Here's how the part is built. I have some questions about the finished solid (model axes, mm). A direction names the side the tool comes from. Give positions to 0.01 mm unless a question says otherwise; leave off trailing zeros. Write each loop counter-clockwise with the first axis right and the second up, starting at its lowest first coordinate (ties: lowest second). Pieces come first, ordered by that corner, then holes. Notation, with made-up numbers: (3, -14) -> (53, -14) arc R21 cw to (53, 6) -> close; hole circle Ø5 at (85, -13). An arc over 180 degrees is marked (long way). Use CSV: the item, a comma, the result in double quotes. Start each with the question number.
(1) Suppose I cut it at A-A on z = 0. List the corners of the cut face in (x, y) for me.
(2) Suppose I cut it at B-B on y = 17. List the corners of the cut face in (x, z) for me.
(3) Suppose I cut it at D-D on z = 72.5. List the corners of the cut face in (x, y) for me, plus the area to 3 significant figures.
(4) For pin 1 Ø3 at (x, z) = (2, -11) entering from +Y; pin 2 Ø8 at (x, y) = (-5, -31) entering from +Z; pin 3 Ø8 at (x, y) = (-2.5, -30.5) entering from +Z; pin 4 Ø10 at (y, z) = (-3, 69) entering from +X, each with a flat end and sliding along its axis, tell me the tip position at first contact or that it passes through.
(5) I need wall thicknesses on L1, parallel to Z at x = -6.05, y = 0; L2, parallel to X at y = 20.5, z = 6. Which ranges of each line are inside material? Lowest first, please. Write a range as [from, to].
(6) If we mould it in two halves opening along X, with no side actions, what happens to faces 5 (the flat face through (-7, 28, 28)), 6 (the flat face through (0.035, -1.003, 85.533)), 7 (the cylindrical face through (-5.23, -32.08, 20.46))? For each: pulls with the +X half, pulls with the -X half, needs draft (parallel to the pull), parting line crosses it, or undercut.
(7) Which directions (+Z, -Z, +X, -X, +Y, -Y) give clear straight access to the entire face, cutting with the end or side of a thin tool? Please do faces 1 (the flat face through (7, 28, 28)), 2 (the cylindrical face through (-0.54, -2.44, 76.39)), 3 (the flat face through (-3.5, -1, -1)), 4 (the flat face through (3.5, -1, -1)).
Autodesk Inventor part; units mm, degrees
ref_plane "YZ Plane" through (0, 0, 0) normal (1, 0, 0) x (0, 1, 0)
ref_plane "XZ Plane" through (0, 0, 0) normal (0, 1, 0) x (-1, 0, 0)
ref_plane "XY Plane" through (0, 0, 0) normal (0, 0, 1) x (1, 0, 0)
sketch "Sketch1" plane through (0, 0, 0) normal (0, 1, 0) x (-1, 0, 0)
  line L0 (7, 0) -> (-7, 0) construction
  line L1 (7, 64.5) -> (-7, 64.5)
  line L2 (-7, 64.5) -> (-7, 38.05)
  line L3 (7, 38.05) -> (-7, 38.05)
  line L4 (7, 38.05) -> (7, 64.5)
  line L5 (3.5, 0) -> (-3.5, 0)
  line L6 (-3.5, 0) -> (-3.5, 38.05)
  line L7 (-3.5, 38.05) -> (3.5, 38.05)
  line L8 (3.5, 38.05) -> (3.5, 0)
  line L9 (3.5, 0) -> (-3.5, 38.05) construction
  line L10 (-3.5, 0) -> (3.5, 38.05) construction
  point P0 (0, 19.025)
  point P1 (0, 38.05)
  point P2 (0, 0)
  point P3 (0, 0)
  dimension "Thickness" = 14
  dimension "DiamExt" = 129
  dimension "PipeDiameter" = 76.1
  dimension "d8" = 7
revolve "Revolution1" add sketch "Sketch1" angle 360 about axis through (-7, 0, 0) along (1, 0, 0)
sketch "Sketch3" plane through (0, 0, 0) normal (0, 0, 1) x (1, 0, 0)
  circle A0 centre (0, 0) radius 2.5
  dimension "d9" = 5
sketch "Sketch4" plane through (0, 0, 0) normal (1, 0, 0) x (0, 1, 0)
  line L0 (0, 0) -> (0, 85.5)
  arc A0 (0, 85.5) -> (-0.9974, 85.5714) centre (0, 92.5) ccw
  dimension "d10" = 7
  dimension "d11" = 92.5
  dimension "d14" = 1
sweep "Sweep1" add profiles "Sketch3" path "Sketch4"
equation "\"d8\" = 0.5 * Thickness"
equation "\"d10\" = 0.5 * Thickness"
equation "\"d11\" = 0.5 * DiamExt + 2 * Thickness"
properties part number "CHECK VALVE SWING WAFER 304L DN65" material "304L"
Geometry says:
1,outline,"(-7, -64.5) -> (7, -64.5) -> (7, -38.05) -> (3.5, -38.05) -> (3.5, 38.05) -> (7, 38.05) -> (7, 64.5) -> (-7, 64.5) -> (-7, 38.05) -> (-3.5, 38.05) -> (-3.5, -38.05) -> (-7, -38.05) -> close"
2,outline,"(-7, -62.22) -> (7, -62.22) -> (7, -34.04) -> (3.5, -34.04) -> (3.5, 34.04) -> (7, 34.04) -> (7, 62.22) -> (-7, 62.22) -> (-7, 34.04) -> (-3.5, 34.04) -> (-3.5, -34.04) -> (-7, -34.04) -> close"
3,outline,"circle Ø5 at (0, 0)"
3,area,"19.6 mm²"
4,pin 1,"y = 63.8"
4,pin 2,"z = 58.58"
4,pin 3,"z = 58.8"
4,pin 4,"x = 7"
5,L1,"[-64.5, -38.05], [38.05, 64.5]"
5,L2,"[-3.5, 3.5]"
6,face 5,"pulls with the -X half"
6,face 6,"undercut"
6,face 7,"needs draft"
7,face 1,"+Z, -Z, +X, +Y, -Y"
7,face 2,"none"
7,face 3,"-X"
7,face 4,"+X"
